```python
from build123d import *

# Parameters (mm, degrees)
SKETCH1_W           = 215.9
SKETCH1_H           = 215.9
SKETCH1_R           = 2.5
SKETCH1_R_2         = 5.08
SKETCH1_R_3         = 44.45
BOSS_EXTRUDE1_DEPTH = 4.7498


with BuildPart() as part:
    # Sketch1 → Boss-Extrude1 (new body)
    with BuildSketch(Plane(origin=(0, 0, 0), x_dir=(1, 0, 0), z_dir=(0, 1, 0))):
        Rectangle(SKETCH1_W, SKETCH1_H)
        with Locations(Location((95.490778515, -95.490778515, 0), (0, 0, 270))):
            Circle(SKETCH1_R, mode=Mode.SUBTRACT)
        with Locations(Location((102.561846327, -102.561846327, 0), (0, 0, 270))):
            Circle(SKETCH1_R, mode=Mode.SUBTRACT)
        with Locations(Location((-95.490778515, -95.490778515, 0), (0, 0, 270))):
            Circle(SKETCH1_R, mode=Mode.SUBTRACT)
        with Locations(Location((-102.561846327, -102.561846327, 0), (0, 0, 270))):
            Circle(SKETCH1_R, mode=Mode.SUBTRACT)
        with Locations(Location((-95.490778515, 95.490778515, 0), (0, 0, 270))):
            Circle(SKETCH1_R, mode=Mode.SUBTRACT)
        with Locations(Location((-102.561846327, 102.561846327, 0), (0, 0, 270))):
            Circle(SKETCH1_R, mode=Mode.SUBTRACT)
        with Locations(Location((95.490778515, 95.490778515, 0), (0, 0, 270))):
            Circle(SKETCH1_R, mode=Mode.SUBTRACT)
        with Locations(Location((102.561846327, 102.561846327, 0), (0, 0, 270))):
            Circle(SKETCH1_R, mode=Mode.SUBTRACT)
        with Locations(Location((86.510522394, -86.510522394, 0), (0, 0, 270))):
            Circle(SKETCH1_R_2, mode=Mode.SUBTRACT)
        with Locations(Location((-86.510522394, -86.510522394, 0), (0, 0, 270))):
            Circle(SKETCH1_R_2, mode=Mode.SUBTRACT)
        with Locations(Location((-86.510522394, 86.510522394, 0), (0, 0, 270))):
            Circle(SKETCH1_R_2, mode=Mode.SUBTRACT)
        with Locations(Location((86.510522394, 86.510522394, 0), (0, 0, 270))):
            Circle(SKETCH1_R_2, mode=Mode.SUBTRACT)
        with Locations(Location((0, 0, 0), (0, 0, 270))):
            Circle(SKETCH1_R_3, mode=Mode.SUBTRACT)
    extrude(amount=BOSS_EXTRUDE1_DEPTH)


solid = part.part
```
Can you work these out from the model? Positions are in its coordinate system, mm. Round coordinates to 2 decimals unless told otherwise and drop trailing zeros. Loops run counter-clockwise (first coordinate to the right, second up) from the corner with the lowest first, then second, coordinate; pieces in that order, holes last. Notation, with made-up numbers: M 20.25,9 L 32.25,9 A15 ccw 32.25,23 Z; hole C 3.5,14 d3. An arc over 180 degrees is marked long. Write item = value, one per line. Start each with the question number.
(1) Suppose I cut it at A-A on z = 0. Write out the boundary of the cut face in (x, y), plus the area to 3 significant figures.
(2) I need wall thicknesses on line 1 along X through (y, z) = (2.5, -95); line 2 along X through (y, z) = (0.5, -86); line 3 along Z through (x, y) = (5, 3.95). Which ranges of each line are inside material? Lowest first, please.
(3) I'm going to push a flat-ended pin straight in: P1, Ø1.5, axis at x = 82, z = 8, coming from the -Y side. Where does the tip first touch, or does it pass through?
(4) Suppose I cut it at B-B on x = 0. Write out the boundary of the cut face in (y, z).
(5) Suppose I cut it at C-C on y = 2.25. Give the number of separate pieces and of enclosed holes in the cut face, plus the area to 3 significant figures.
Answer block:
q1.outline = M -107.95,0 L -44.45,0 L -44.45,4.75 L -107.95,4.75 Z; M 44.45,0 L 107.95,0 L 107.95,4.75 L 44.45,4.75 Z
q1.area = 603 mm²
q2.line_1 = -107.95 to -97.94, -93.04 to 93.04, 97.94 to 107.95
q2.line_2 = -107.95 to -91.56, -81.46 to 81.46, 91.56 to 107.95
q2.line_3 = -107.95 to -44.17, 44.17 to 107.95
q3.P1 = 0
q4.outline = M 0,-107.95 L 4.75,-107.95 L 4.75,-44.45 L 0,-44.45 Z; M 0,44.45 L 4.75,44.45 L 4.75,107.95 L 0,107.95 Z
q5.separate_pieces = 1
q5.enclosed_holes = 13
q5.area = 39,900 mm²
